Answer from the drawing. Dimensions are ordinates in mm from the lowest x, y and z of the part. A direction names the side the tool comes from. Coordinates: 2 decimals unless noted, no trailing zeros. Order: outer loops, then holes, each group sorted by start corner. A loop starts at its lowest first (then second) coordinate and runs counter-clockwise, first axis right, second up. Notation, with made-up numbers: (-23.75, 10) - (11.25, 10) arc R23 cw to (11.25, 29) - close; hole circle Ø6 at (7.25, 42). An arc over 180 degrees is marked (long way). Use a Markdown table: item, result. Add a question column.
Item 1: The part is cut by section B-B, the plane y = 10.25. Give the vertices of the cut face in (x, z).
Item 2: The part is cut by section A-A, the plane x = 10.25. Give the vertices of the cut face in (y, z), then the cut area to 4 significant figures.
Item 3: The part is cut by section D-D, the plane z = 5.5. Give the vertices of the cut face in (x, y).
Item 4: Flat-ended cylindrical pins translate along their axes: P1, Ø3, axis at y = 8.5, z = 1.5, coming from the -X side; P2, Ø1.5, axis at x = 4.5, z = 4, coming from the -Y side. Find the tip coordinate at first contact, or state that the pin passes through.
Item 5: The mould has two halves that part along Y. Classify the marked faces 4, 5 and 6: released by +Y, released by -Y, zero draft, split by the parting line, or undercut.
Item 6: Find the intervals of material crossed by line 1 along Y through (x, z) = (10.25, 6.45); line 2 along Z through (x, y) = (12.25, 15); line 3 along Y through (x, z) = (6.25, 2.5), in increasing order.
Item 7: The part is cut by section C-C, the plane z = 1. Give the vertices of the cut face in (x, y).
Item 8: For the marked faces 1, 2 and 3, determine the directions among +Z, -Z, +X, -X, +Y, -Y from which every point of the face is accessible in a straight line to the end or side of a thin tool.
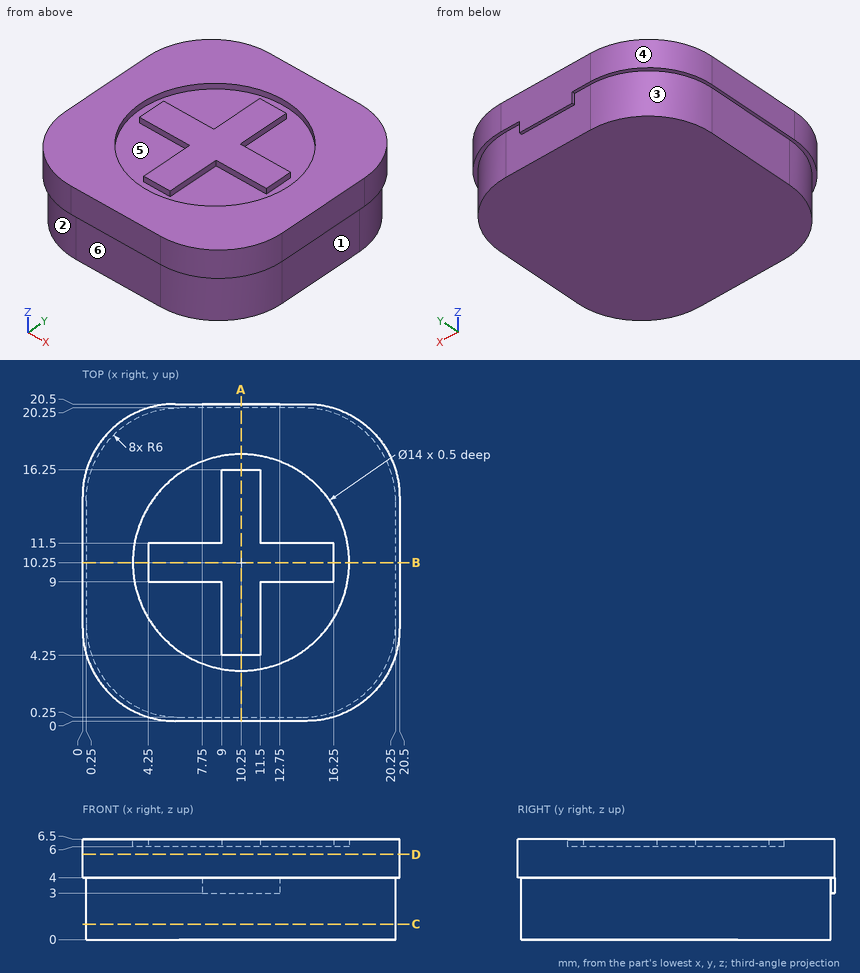
Solution:
| question | item | result |
|---|---|---|
| 1 | outline | (0, 4) - (0.25, 4) - (0.25, 0) - (20.25, 0) - (20.25, 4) - (20.5, 4) - (20.5, 6.5) - (17.25, 6.5) - (17.25, 6) - (16.25, 6) - (16.25, 6.5) - (4.25, 6.5) - (4.25, 6) - (3.25, 6) - (3.25, 6.5) - (0, 6.5) - close |
| 2 | outline | (0, 4) - (0.25, 4) - (0.25, 0) - (20.25, 0) - (20.25, 3) - (20.5, 3) - (20.5, 6.5) - (17.25, 6.5) - (17.25, 6) - (16.25, 6) - (16.25, 6.5) - (4.25, 6.5) - (4.25, 6) - (3.25, 6) - (3.25, 6.5) - (0, 6.5) - close |
| 2 | area | 130.5 mm2 |
| 3 | outline | (0, 6) arc R6 ccw to (6, 0) - (14.5, 0) arc R6 ccw to (20.5, 6) - (20.5, 14.5) arc R6 ccw to (14.5, 20.5) - (6, 20.5) arc R6 ccw to (0, 14.5) - close |
| 4 | P1 | stops at x = 0.25 |
| 4 | P2 | stops at y = 0.05 |
| 5 | face 4 | released by +Y |
| 5 | face 5 | undercut |
| 5 | face 6 | released by -Y |
| 6 | line 1 | y = 0 to 3.25, 4.25 to 16.25, 17.25 to 20.5 |
| 6 | line 2 | z = 0 to 6 |
| 6 | line 3 | y = 0.25 to 20.25 |
| 7 | outline | (0.25, 6.25) arc R6 ccw to (6.25, 0.25) - (14.25, 0.25) arc R6 ccw to (20.25, 6.25) - (20.25, 14.25) arc R6 ccw to (14.25, 20.25) - (6.25, 20.25) arc R6 ccw to (0.25, 14.25) - close |
| 8 | face 1 | -Z, +X, +Y, -Y |
| 8 | face 2 | -Z, -X, -Y |
| 8 | face 3 | -Z, -X, +Y |
